```python
from build123d import *

# Parameters (mm, degrees)
SKETCH1_R                = 72.5
BOSS_EXTRUDE1_DEPTH      = 294
FILLET1_R                = 72.5
SKETCH2_R                = 63.5
BOSS_EXTRUDE2_DEPTH      = 584.2
BOSS_EXTRUDE3_DEPTH      = 78
BOSS_EXTRUDE3_DEPTH_BACK = 85.75
SKETCH3_R                = 67
CHAMFER1_SIZE            = 5
CHAMFER2_SIZE            = 7
CHAMFER2_SIZE2           = 16
SHELL1_3_OUTLINE_W       = 53.5
SHELL1_3_OUTLINE_H       = 532.228338498


with BuildPart() as part:
    # Sketch1 → Boss-Extrude1 (new body)
    with BuildSketch(Plane.XY):
        Circle(SKETCH1_R)
    extrude(amount=BOSS_EXTRUDE1_DEPTH)

    # Fillet1
    fillet1_edges = [part.edges().sort_by_distance(p)[0] for p in [
        (-72.5, 0, 294),
    ]]
    fillet(fillet1_edges, radius=FILLET1_R)

    # Sketch2 → Boss-Extrude2 (add)
    with BuildSketch(Plane(origin=(0, 0, 0), x_dir=(1, 0, 0), z_dir=(0, 1, 0))):
        with Locations(Location((0, -85.5, 0), (0, 0, 270))):
            Circle(SKETCH2_R)
    extrude(amount=-BOSS_EXTRUDE2_DEPTH)

    # Sketch3 → Boss-Extrude3 (add, two sides: drawn at the far end of the back side and taken through both)
    with BuildSketch(Plane.XY.offset(85.5).offset(-BOSS_EXTRUDE3_DEPTH_BACK)):
        with Locations((0, -584.2)):
            Circle(SKETCH3_R)
    extrude(amount=BOSS_EXTRUDE3_DEPTH + BOSS_EXTRUDE3_DEPTH_BACK)

    # Chamfer1
    chamfer1_edges = [part.edges().sort_by_distance(p)[0] for p in [
        (-67, -584.2, 163.5),
    ]]
    chamfer(chamfer1_edges, length=CHAMFER1_SIZE)

    # Chamfer2
    chamfer2_edges = [part.edges().sort_by_distance(p)[0] for p in [
        (-67, -584.2, -0.25),
    ]]
    chamfer2_side = [part.faces().sort_by_distance(p)[0] for p in [
        (0, -584.2, -0.25),
    ]]
    chamfer(chamfer2_edges, length=CHAMFER2_SIZE, length2=CHAMFER2_SIZE2, reference=chamfer2_side[0])

    # Sketch4 → Cut-Revolve1 (revolve, cut)
    with BuildSketch(Plane(origin=(0, 0, 0), x_dir=(1, 0, 0), z_dir=(0, 1, 0)), mode=Mode.PRIVATE) as cut_revolve1_sk:
        with BuildLine():
            Line((81.109243283, -151.148251361), (72.5, -151.148251361))
            Line((72.5, -151.148251361), (72.5, -171.148251361))
            Line((72.5, -171.148251361), (57.5, -186.148251361))
            Line((57.5, -186.148251361), (57.5, -201.148251361))
            Line((57.5, -201.148251361), (49.5, -209.148251361))
            ThreePointArc((49.5, -209.148251361), (35.001785669, -244.15003703), (0, -258.648251361))
            Line((0, -258.648251361), (0, -319.881343941))
            Line((0, -319.881343941), (156.304849296, -319.881343941))
            Line((156.304849296, -319.881343941), (156.304849296, -151.148251361))
            Line((156.304849296, -151.148251361), (81.109243283, -151.148251361))
        make_face()
    revolve(cut_revolve1_sk.sketch.rotate(Axis((0, 0, 258.648251361), (0, 0, 1)), 180), axis=Axis((0, 0, 258.648251361), (0, 0, 1)), mode=Mode.SUBTRACT)

    # Shell1: read off the stored shape, not the designer's step
    # Shell1 outline → Shell1 (revolve, cut)
    with BuildSketch(Plane.XZ.offset(584.2)):
        Polygon((49.084844252, -0.25), (57, 17.841784567), (57, 153.5), (0, 153.5), (0, -0.25), align=None)
    revolve(axis=Axis((0, -584.2, 0), (0, 0, 1)), mode=Mode.SUBTRACT)

    # Shell1 2 outline → Shell1 2 (revolve, cut)
    with BuildSketch(Plane.XZ):
        with BuildLine():
            Line((62.5, 0), (62.5, 167.006115737))
            Line((62.5, 167.006115737), (47.5, 182.006115737))
            Line((47.5, 182.006115737), (47.5, 197.006115737))
            Line((47.5, 197.006115737), (39.302538652, 205.203577042))
            ThreePointArc((39.302538652, 205.203577042), (29.292188682, 235.647641584), (0, 248.648251361))
            Line((0, 248.648251361), (0, 0))
            Line((0, 0), (62.5, 0))
        make_face()
    revolve(axis=Axis((0, 0, 0), (0, 0, 1)), mode=Mode.SUBTRACT)

    # Shell1 3 outline → Shell1 3 (revolve, cut)
    with BuildSketch(Plane.XY.offset(85.5)):
        with Locations((26.75, -298.423797413)):
            Rectangle(SHELL1_3_OUTLINE_W, SHELL1_3_OUTLINE_H)
    revolve(axis=Axis((0, 0, 85.5), (0, 1, 0)), mode=Mode.SUBTRACT)


solid = part.part
```
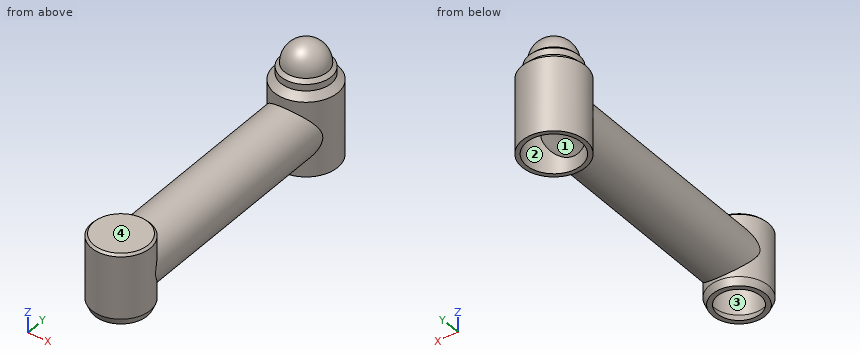
CAD build for the part. Positions are in the model's coordinates, mm. Face numbers are marked on the shaded views. A direction names the side the tool comes from. Coordinates: 2 decimals unless noted, no trailing zeros. Loops run counter-clockwise (first coordinate to the right, second up) from the corner with the lowest first, then second, coordinate; pieces in that order, holes last. Notation, with made-up numbers: (27, -7.75) - (52, -7.75) arc R23 ccw to (52, 25.25) - close; hole circle Ø1 at (85, -8). An arc over 180 degrees is marked (long way). Return JSON: item names as keys, results as strings.
1. Band-saw the part on D-D (z = 127). Give the cut face in (x, y).
Result:
{"outline": "(-48.06, -537.52) arc R67 ccw (long way) to (48.06, -537.52) - (48.06, -54.28) arc R72.5 ccw (long way) to (-48.06, -54.28) - close; hole (-33.76, -538.28) arc R57 ccw (long way) to (33.76, -538.28) - (33.76, -52.6) arc R62.5 ccw (long way) to (-33.76, -52.6) - close"}
2. 3-axis set-ups, long thin cutter, end or side, ignore diameter. For the marked faces 1 and 2: which of +Z, -Z, +X, -X, +Y, -Y reach the whole face in a straight line?
Result:
{"face 1": "none", "face 2": "-Z"}
3. Band-saw the part on C-C (y = 0). Give the cut face in (x, z), and give its area (3 significant figures).
Result:
{"outline": "(-72.5, 0) - (-62.5, 0) - (-62.5, 167.01) - (-47.5, 182.01) - (-47.5, 197.01) - (-39.3, 205.2) arc R39.5 cw (long way) to (39.3, 205.2) - (47.5, 197.01) - (47.5, 182.01) - (62.5, 167.01) - (62.5, 0) - (72.5, 0) - (72.5, 171.15) - (57.5, 186.15) - (57.5, 201.15) - (49.5, 209.15) arc R49.5 ccw to (-49.5, 209.15) - (-57.5, 201.15) - (-57.5, 186.15) - (-72.5, 171.15) - close", "area": "5,770 mm2"}
4. Band-saw the part on B-B (y = -241.5). Give the cut face in (x, z).
Result:
{"outline": "circle Ø127 at (0, 85.5); hole circle Ø107 at (0, 85.5)"}
5. Mould opens along Y. For the marked faces 3 and 4 say: released by +Y, released by -Y, zero draft, split by the parting line, or undercut.
Result:
{"face 3": "undercut", "face 4": "zero draft"}
6. Band-saw the part on A-A (z = 85.5). Give the cut face in (x, y).
Result:
{"outline": "(-63.5, -562.83) arc R67 ccw (long way) to (63.5, -562.83) - (63.5, -34.99) arc R72.5 ccw (long way) to (-63.5, -34.99) - close; hole (-53.5, -564.53) arc R57 ccw (long way) to (53.5, -564.53) - (53.5, -32.31) arc R62.5 ccw (long way) to (-53.5, -32.31) - close"}
7. Probe L1, parallel to Y at x = 0, z = 190; L2, parallel to Z at x = 0, y = -176; L3, parallel to Y at x = 0, z = 111. List the from-to ranges inside material, lowest first. Write a range as from..to.
Result:
{"L1": "y = -57.5..-47.5, 47.5..57.5", "L2": "z = 22..32, 139..149", "L3": "y = -651.2..-641.2, 62.5..72.5"}
8. Drop flat-ended pins along their axis: pin 1 (12 mm diameter, centred on x = 12, z = 216, fed in from +Y); pin 2 (12 mm diameter, centred on x = -5, y = -566, fed in from -Z); pin 3 (2 mm diameter, centred on x = -33.5, z = 106, fed in from -Y). Give the stop position or say it passes through.
Result:
{"pin 1": "stops at y = 48.88", "pin 2": "stops at z = 153.5", "pin 3": "stops at y = -642.79"}
